from build123d import *

# Parameters (mm, degrees)
SKETCH1_R           = 1.75
BOSS_EXTRUDE1_DEPTH = 1.5


with BuildPart() as part:
    # Sketch1 → Boss-Extrude1 (new body)
    # profile 1 of 3: a face of its own
    with BuildSketch(Plane.XY):
        Polygon((44, 0), (0, 0), (1.563260572, -5.210868574), (3, -10), (44, -10), align=None)
    # profile 2 of 3: a face of its own
    with BuildSketch(Plane.XY):
        Polygon((1.563260572, 5.210868574), (0, 0), (44, 0), (44, 10), (3, 10), align=None)
    # profile 3 of 3: a face of its own
    with BuildSketch(Plane.XY):
        with BuildLine():
            Line((1.563260572, -5.210868574), (0, 0))
            Line((0, 0), (1.563260572, 5.210868574))
            Line((1.563260572, 5.210868574), (-6.388542044, 5.210868574))
            ThreePointArc((-6.388542044, 5.210868574), (-11.194271022, 10), (-16, 5.210868574))
            Line((-16, 5.210868574), (-16, -5.210868574))
            ThreePointArc((-16, -5.210868574), (-11.194271022, -10), (-6.388542044, -5.210868574))
            Line((-6.388542044, -5.210868574), (1.563260572, -5.210868574))
        make_face()
        with Locations((-11.260632468, -7)):
            Circle(SKETCH1_R, mode=Mode.SUBTRACT)
        with Locations((-11.260632468, 7)):
            Circle(SKETCH1_R, mode=Mode.SUBTRACT)
    extrude(amount=BOSS_EXTRUDE1_DEPTH)


solid = part.part
Work out the finished part from the listing and answer in its coordinate system (mm). A direction names the side the tool comes from. Round coordinates to 2 decimals unless told otherwise and drop trailing zeros. Loops run counter-clockwise (first coordinate to the right, second up) from the corner with the lowest first, then second, coordinate; pieces in that order, holes last. Notation, with made-up numbers: (6, 29.25) - (27, 29.25) arc R17 ccw to (27, 58.25) - close; hole circle Ø11 at (-23, 78). An arc over 180 degrees is marked (long way). One line per item, written item: value.
Q1. Find section C-C on x = 1. Give the vertices of the cut face in (y, z), and give its area (3 significant figures).
Check values:
outline: (-5.21, 0) - (5.21, 0) - (5.21, 1.5) - (-5.21, 1.5) - close
area: 15.6 mm2
Q2. Find section A-A on z = 1.1. Give the vertices of the cut face in (x, y), and give its area (3 significant figures).
Check values:
outline: (-16, -5.21) arc R4.81 ccw to (-6.39, -5.21) - (1.56, -5.21) - (3, -10) - (44, -10) - (44, 10) - (3, 10) - (1.56, 5.21) - (-6.39, 5.21) arc R4.81 ccw to (-16, 5.21) - close; hole circle Ø3.5 at (-11.26, -7); hole circle Ø3.5 at (-11.26, 7)
area: 1,080 mm2
Q3. Straight lines are drawn through the part: probe 1 along X at (y, z) = (-7.75, 1.1) (1 decimal); probe 2 along Y at (x, z) = (-2, 1.15); probe 3 along Y at (x, z) = (-11, 1.35). For each, find the intervals that lie inside material, in ascending order.
Check values:
probe 1: -15.3 to -12.8, -9.7 to -7.1, 2.3 to 44
probe 2: -5.21 to 5.21
probe 3: -10 to -8.73, -5.27 to 5.27, 8.73 to 10
Q4. Find section B-B on y = -7. Give the vertices of the cut face in (x, z).
Check values:
outline: (-15.65, 0) - (-13.01, 0) - (-13.01, 1.5) - (-15.65, 1.5) - close; (-9.51, 0) - (-6.74, 0) - (-6.74, 1.5) - (-9.51, 1.5) - close; (2.1, 0) - (44, 0) - (44, 1.5) - (2.1, 1.5) - close
Q5. For faces 1 (the cylindrical face through (-10.45, -8.55, 0.74)), 2 (the flat face through (2.29, 7.64, 0.74)), 3 (the flat face through (2.27, -7.57, 0.74)), determine the directions among +Z, -Z, +X, -X, +Y, -Y from which every point of the face is accessible in a straight line to the end or side of a thin tool.
Check values:
face 1: +Z, -Z
face 2: +Z, -Z, +Y
face 3: +Z, -Z, -Y
Q6. The mould has two halves that part along X. Classify faces 4 (the cylindrical face through (-10.45, 5.45, 0.74)), 5 (the flat face through (-16, 0, 1)), 6 (the flat face through (23, -10, 1)), 7 (the flat face through (-2, 5.211, 1)): +X half, -X half, draft (parallel to the pull), parting line (faces both ways), or undercut.
Check values:
face 4: undercut
face 5: -X half
face 6: draft
face 7: undercut
